Source: CAD feature listing. Evaluate the final solid. Frame: model axes, mm. Face numbers are marked on the shaded views. A direction names the side the tool comes from. Round coordinates to 2 decimals unless told otherwise and drop trailing zeros. Write each loop counter-clockwise with the first axis right and the second up, starting at its lowest first coordinate (ties: lowest second). Pieces come first, ordered by that corner, then holes.
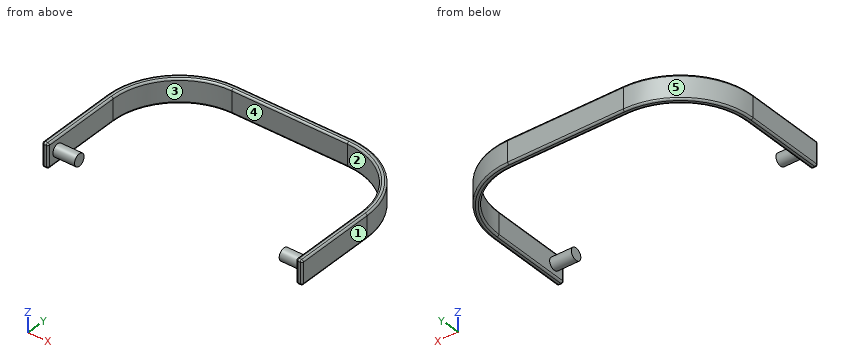
```python
from build123d import *

# Parameters (mm, degrees)
SKETCH_2_W               = 216
SKETCH_2_H               = 128
EXTRUDE_1_DEPTH          = 20
FILLET_1_R               = 60
CUT_EXTRUDE_1_DEPTH      = 252.872983863
CUT_EXTRUDE_1_DEPTH_BACK = 20
SKETCH_4_R               = 5
EXTRUDE_2_DEPTH          = 18
EXTRUDE_START            = 18
SKETCH_5_R               = 5
EXTRUDE_3_DEPTH          = 18
FILLET_2_R               = 1.5


with BuildPart() as part:
    # ｽｹｯﾁ2 → ﾎﾞｽ - 押し出し1 (new body)
    with BuildSketch(Plane.XY):
        with Locations((108, 64)):
            Rectangle(SKETCH_2_W, SKETCH_2_H)
    extrude(amount=EXTRUDE_1_DEPTH)

    # ﾌｨﾚｯﾄ1
    fillet_1_edges = [part.edges().sort_by_distance(p)[0] for p in [
        (0, 128, 10),
        (216, 128, 10),
    ]]
    fillet(fillet_1_edges, radius=FILLET_1_R)

    # ｽｹｯﾁ3 → ｶｯﾄ - 押し出し1 (cut, two sides: drawn at the far end of the back side and taken through both)
    with BuildSketch(Plane.XY.offset(20).offset(-CUT_EXTRUDE_1_DEPTH_BACK)):
        with BuildLine():
            Line((211, -503.578767777), (211, 0))
            Line((211, 0), (211, 68))
            ThreePointArc((211, 68), (194.890872965, 106.890872965), (156, 123))
            Line((156, 123), (60, 123))
            ThreePointArc((60, 123), (21.109127035, 106.890872965), (5, 68))
            Line((5, 68), (5, 0))
            Line((5, 0), (5, -503.578767777))
            Line((5, -503.578767777), (5, -1510.73630333))
            Line((5, -1510.73630333), (211, -1510.73630333))
            Line((211, -1510.73630333), (211, -503.578767777))
        make_face()
    extrude(amount=CUT_EXTRUDE_1_DEPTH + CUT_EXTRUDE_1_DEPTH_BACK, mode=Mode.SUBTRACT)

    # ｽｹｯﾁ4 → ﾎﾞｽ - 押し出し2 (add)
    with BuildSketch(Plane(origin=(5, 0, 0), x_dir=(0, 0, -1), z_dir=(1, 0, 0))):
        with Locations(Location((-10, 10, 0), (0, 0, 270))):
            Circle(SKETCH_4_R)
    extrude(amount=EXTRUDE_2_DEPTH)

    # ｽｹｯﾁ5 → ﾎﾞｽ - 押し出し3 (add)
    with BuildSketch(Plane.ZY.offset(-211).offset(EXTRUDE_START)):
        with Locations(Location((10, 10, 0), (0, 0, 270))):
            Circle(SKETCH_5_R)
    extrude(amount=-EXTRUDE_3_DEPTH)

    # ﾌｨﾚｯﾄ2
    fillet_2_edges = [part.edges().sort_by_distance(p)[0] for p in [
        (216, 34, 20),
        (108, 128, 0),
        (108, 128, 20),
        (0, 34, 0),
        (17.573593129, 110.426406871, 0),
        (198.426406871, 110.426406871, 0),
        (0, 34, 20),
        (17.573593129, 110.426406871, 20),
        (198.426406871, 110.426406871, 20),
        (213.5, 0, 0),
        (213.5, 0, 20),
        (211, 0, 10),
        (211, 34, 20),
        (194.890872965, 106.890872965, 20),
        (108, 123, 20),
        (21.109127035, 106.890872965, 20),
        (5, 34, 20),
        (5, 0, 10),
        (5, 34, 0),
        (211, 34, 0),
        (194.890872965, 106.890872965, 0),
        (108, 123, 0),
        (21.109127035, 106.890872965, 0),
        (216, 34, 0),
        (2.5, 0, 0),
        (216, 0, 10),
        (0, 0, 10),
        (2.5, 0, 20),
    ]]
    fillet(fillet_2_edges, radius=FILLET_2_R)


solid = part.part
```
Q1. Section query B-B, the plane z = 10. Output: boundary loops of the cut face in (x, y).
Q2. Line query: line 1 (X direction, y = 30, z = 16.5); line 2 (Y direction, x = 87, z = 2.5); line 3 (X direction, y = 81, z = 15). Output: solid intervals per line, ascending.
Q3. Pin query (flat end, axial travel): P1, Ø2, axis at x = 189, z = 9, coming from the -Y side; P2, Ø10, axis at x = 157, z = 3.5, coming from the -Y side; P3, Ø5, axis at x = 26.5, z = 2, coming from the -Y side. Return the tip coordinate at first contact, or that it passes through.
Q4. Mould query, pull axis Y, two halves, no side actions, for the marked faces 3, 4 and 5. Classes: pulls with the +Y half, pulls with the -Y half, needs draft (parallel to the pull), parting line crosses it, or undercut.
Q5. Section query C-C, the plane x = 83.5. Output: boundary loops of the cut face in (y, z), and give its area (3 significant figures).
Q6. Set-up query: the marked faces 1 and 2. Return all of +Z, -Z, +X, -X, +Y, -Y with unobstructed straight access to the full face (end or side cutting, diameter ignored); none if empty.
Q7. Section query A-A, the plane y = 10. Output: boundary loops of the cut face in (x, z).
Filled in:
1. outline: (0, 1.5) arc R1.5 ccw to (1.5, 0) - (3.5, 0) arc R1.5 ccw to (5, 1.5) - (5, 5) - (23, 5) - (23, 15) - (5, 15) - (5, 68) arc R55 cw to (60, 123) - (156, 123) arc R55 cw to (211, 68) - (211, 15) - (193, 15) - (193, 5) - (211, 5) - (211, 1.5) arc R1.5 ccw to (212.5, 0) - (214.5, 0) arc R1.5 ccw to (216, 1.5) - (216, 68) arc R60 ccw to (156, 128) - (60, 128) arc R60 ccw to (0, 68) - close
2. line 1: x = 0 to 5, 211 to 216
2. line 2: y = 123 to 128
2. line 3: x = 1.43 to 6.56, 209.44 to 214.57
3. P1: stops at y = 111.23
3. P2: stops at y = 122.67
3. P3: stops at y = 109.58
4. face 3: undercut
4. face 4: pulls with the -Y half
4. face 5: pulls with the +Y half
5. outline: (123, 1.5) arc R1.5 ccw to (124.5, 0) - (126.5, 0) arc R1.5 ccw to (128, 1.5) - (128, 18.5) arc R1.5 ccw to (126.5, 20) - (124.5, 20) arc R1.5 ccw to (123, 18.5) - close
5. area: 98.1 mm2
6. face 1: +Z, -Z, +X, +Y, -Y
6. face 2: +Z, -Z
7. outline: (0, 1.5) arc R1.5 ccw to (1.5, 0) - (3.5, 0) arc R1.5 ccw to (5, 1.5) - (5, 5) - (23, 5) - (23, 15) - (5, 15) - (5, 18.5) arc R1.5 ccw to (3.5, 20) - (1.5, 20) arc R1.5 ccw to (0, 18.5) - close; (193, 5) - (211, 5) - (211, 1.5) arc R1.5 ccw to (212.5, 0) - (214.5, 0) arc R1.5 ccw to (216, 1.5) - (216, 18.5) arc R1.5 ccw to (214.5, 20) - (212.5, 20) arc R1.5 ccw to (211, 18.5) - (211, 15) - (193, 15) - close
